```python
from build123d import *

# Parameters (mm, degrees)
SKETCH_1_W                     = 52
SKETCH_1_H                     = 44
EXTRUDE_1_DEPTH                = 7
SKETCH_2_W                     = 40.4
SKETCH_2_H                     = 40.4
CUT_EXTRUDE_1_DEPTH            = 5.5
SKETCH_4_W                     = 7.08
SKETCH_4_H                     = 40.4
EXTRUDE_2_DEPTH                = 1
SKETCH_5_W                     = 5.8
SKETCH_5_H                     = 25.6
CUT_EXTRUDE_2_DEPTH            = 1
SKETCH_7_R                     = 1
CUT_EXTRUDE_3_DEPTH            = 63.531991812
EXTRUDE_3_REACH                = 64.682
SKETCH_13_R                    = 1.75
HOLE_WIZARD_M1_6_1_D           = 1.8
HOLE_WIZARD_M1_6_1_CBORE_D     = 2.6
HOLE_WIZARD_M1_6_1_CBORE_DEPTH = 0.8
CHAMFER_1_SIZE                 = 5.5
CUT_EXTRUDE_4_DEPTH            = 1.6
SKETCH_15_W                    = 10
SKETCH_15_H                    = 12.713519239
CUT_EXTRUDE_5_DEPTH            = 5
CHAMFER_2_SIZE                 = 0.6
FILLET_1_R                     = 1
SKETCH_19_R                    = 0.9
CUT_EXTRUDE_9_DEPTH            = 1.6


with BuildPart() as part:
    # 스케치1 → 보스-돌출1 (new body)
    with BuildSketch(Plane(origin=(0, 7, 0), x_dir=(1, 0, 0), z_dir=(0, 1, 0))):
        with Locations((20, 20)):
            Rectangle(SKETCH_1_W, SKETCH_1_H)
    extrude(amount=-EXTRUDE_1_DEPTH)

    # 스케치2 → 컷-돌출1 (cut)
    with BuildSketch(Plane.XZ):
        with Locations((20, -20)):
            Rectangle(SKETCH_2_W, SKETCH_2_H)
    extrude(amount=-CUT_EXTRUDE_1_DEPTH, mode=Mode.SUBTRACT)

    # 스케치4 → 보스-돌출2 (add)
    # profile 1 of 2: a face of its own
    with BuildSketch(Plane.XZ.offset(-5.5)):
        with Locations((3.34, -20)):
            Rectangle(SKETCH_4_W, SKETCH_4_H)
        with BuildLine():
            Line((4.64, -5), (4.64, -15))
            ThreePointArc((4.64, -15), (3.34, -16.3), (2.04, -15))
            Line((2.04, -15), (2.04, -5))
            ThreePointArc((2.04, -5), (3.34, -3.7), (4.64, -5))
        make_face(mode=Mode.SUBTRACT)
        with BuildLine():
            Line((4.64, -25), (4.64, -35))
            ThreePointArc((4.64, -35), (3.34, -36.3), (2.04, -35))
            Line((2.04, -35), (2.04, -25))
            ThreePointArc((2.04, -25), (3.34, -23.7), (4.64, -25))
        make_face(mode=Mode.SUBTRACT)
    # profile 2 of 2: a face of its own
    with BuildSketch(Plane.XZ.offset(-5.5)):
        with Locations((36.66, -20)):
            Rectangle(SKETCH_4_W, SKETCH_4_H)
        with BuildLine():
            Line((37.96, -5), (37.96, -15))
            ThreePointArc((37.96, -15), (36.66, -16.3), (35.36, -15))
            Line((35.36, -15), (35.36, -5))
            ThreePointArc((35.36, -5), (36.66, -3.7), (37.96, -5))
        make_face(mode=Mode.SUBTRACT)
        with BuildLine():
            Line((35.36, -35), (35.36, -25))
            ThreePointArc((35.36, -25), (36.66, -23.7), (37.96, -25))
            Line((37.96, -25), (37.96, -35))
            ThreePointArc((37.96, -35), (36.66, -36.3), (35.36, -35))
        make_face(mode=Mode.SUBTRACT)
    extrude(amount=EXTRUDE_2_DEPTH)

    # 스케치5 → 컷-돌출2 (cut)
    with BuildSketch(Plane.XZ):
        with Locations((43.1, -20)):
            Rectangle(SKETCH_5_W, SKETCH_5_H)
        with Locations((-3.1, -20)):
            Rectangle(SKETCH_5_W, SKETCH_5_H)
    extrude(amount=-CUT_EXTRUDE_2_DEPTH, mode=Mode.SUBTRACT)

    # 스케치7 → 컷-돌출3 (cut, through all)
    with BuildSketch(Plane.XZ.offset(-5.5)):
        with Locations(Location((28.92, -37.4, 0), (0, 0, 270))):
            Circle(SKETCH_7_R)
        with Locations(Location((11.08, -37.4, 0), (0, 0, 270))):
            Circle(SKETCH_7_R)
    extrude(amount=-CUT_EXTRUDE_3_DEPTH, mode=Mode.SUBTRACT)

    # 스케치13 → 보스-돌출3 (add, up to next)
    with BuildSketch(Plane.XZ, mode=Mode.PRIVATE) as extrude_3_sk1:
        with Locations((7.5, 0)):
            Circle(SKETCH_13_R)
    extrude_3_tool1 = extrude(extrude_3_sk1.sketch, amount=-EXTRUDE_3_REACH, mode=Mode.PRIVATE) - part.part
    # 스케치13 → 보스-돌출3 (add, up to next)
    with BuildSketch(Plane.XZ, mode=Mode.PRIVATE) as extrude_3_sk2:
        with Locations((32.5, 0)):
            Circle(SKETCH_13_R)
    extrude_3_tool2 = extrude(extrude_3_sk2.sketch, amount=-EXTRUDE_3_REACH, mode=Mode.PRIVATE) - part.part
    # 스케치13 → 보스-돌출3 (add, up to next)
    with BuildSketch(Plane.XZ, mode=Mode.PRIVATE) as extrude_3_sk3:
        with Locations((32.5, -40)):
            Circle(SKETCH_13_R)
    extrude_3_tool3 = extrude(extrude_3_sk3.sketch, amount=-EXTRUDE_3_REACH, mode=Mode.PRIVATE) - part.part
    # 스케치13 → 보스-돌출3 (add, up to next)
    with BuildSketch(Plane.XZ, mode=Mode.PRIVATE) as extrude_3_sk4:
        with Locations((7.5, -40)):
            Circle(SKETCH_13_R)
    extrude_3_tool4 = extrude(extrude_3_sk4.sketch, amount=-EXTRUDE_3_REACH, mode=Mode.PRIVATE) - part.part
    add(extrude_3_tool1.solids().sort_by_distance((7.5, 0, 0))[0])
    add(extrude_3_tool2.solids().sort_by_distance((32.5, 0, 0))[0])
    add(extrude_3_tool3.solids().sort_by_distance((32.5, 0, -40))[0])
    add(extrude_3_tool4.solids().sort_by_distance((7.5, 0, -40))[0])

    # M1.6 남비 머리 나사용 카운터보어1 (through all)
    with Locations(Plane(origin=(0, 7, 0), x_dir=(1, 0, 0), z_dir=(0, 1, 0))):
        with Locations((7.5, 0), (32.5, 0), (7.5, 40), (32.5, 40)):
            CounterBoreHole(HOLE_WIZARD_M1_6_1_D / 2, HOLE_WIZARD_M1_6_1_CBORE_D / 2, HOLE_WIZARD_M1_6_1_CBORE_DEPTH)

    # 모따기1
    chamfer_1_edges = [part.edges().sort_by_distance(p)[0] for p in [
        (46, 7, -20),
        (-6, 7, -20),
    ]]
    chamfer(chamfer_1_edges, length=CHAMFER_1_SIZE)

    # 스케치14 → 컷-돌출4 (cut)
    with BuildSketch(Plane.XZ):
        with BuildLine():
            Line((34.238533865, 0.2), (30.761466135, 0.2))
            ThreePointArc((30.761466135, 0.2), (32.5, -1.75), (34.238533865, 0.2))
        make_face()
        with BuildLine():
            Line((9.238533865, 0.2), (5.761466135, 0.2))
            ThreePointArc((5.761466135, 0.2), (7.5, -1.75), (9.238533865, 0.2))
        make_face()
        with BuildLine():
            Line((9.238533865, -40.2), (5.761466135, -40.2))
            ThreePointArc((5.761466135, -40.2), (7.5, -38.25), (9.238533865, -40.2))
        make_face()
        with BuildLine():
            Line((34.238533865, -40.2), (30.761466135, -40.2))
            ThreePointArc((30.761466135, -40.2), (32.5, -38.25), (34.238533865, -40.2))
        make_face()
    extrude(amount=-CUT_EXTRUDE_4_DEPTH, mode=Mode.SUBTRACT)

    # 스케치15 → 컷-돌출5 (cut)
    with BuildSketch(Plane.XZ):
        with Locations((20, -41.191132848)):
            Rectangle(SKETCH_15_W, SKETCH_15_H)
    extrude(amount=-CUT_EXTRUDE_5_DEPTH, mode=Mode.SUBTRACT)

    # 모따기2
    chamfer_2_edges = [part.edges().sort_by_distance(p)[0] for p in [
        (46, 0.75, 2),
        (46, 0.75, -42),
        (-6, 0.75, -42),
        (20, 7, 2),
        (20, 7, -42),
        (-6, 0.75, 2),
    ]]
    chamfer(chamfer_2_edges, length=CHAMFER_2_SIZE)

    # 필렛1
    fillet_1_edges = [part.edges().sort_by_distance(p)[0] for p in [
        (6.88, 5, -1.636490147),
        (9.238533865, 3.55, 0.2),
        (34.238533865, 3.05, 0.2),
        (33.12, 5, -1.636490147),
        (33.12, 5, -38.363509853),
        (30.761466135, 3.55, -40.2),
        (6.88, 5, -38.363509853),
        (5.761466135, 3.05, -40.2),
        (34.238533865, 3.05, -40.2),
        (9.238533865, 3.55, -40.2),
        (30.761466135, 3.55, 0.2),
        (5.761466135, 3.05, 0.2),
        (-0.2, 2.25, -40.2),
        (-0.2, 2.25, 0.2),
        (40.2, 2.25, -40.2),
        (40.2, 2.25, 0.2),
    ]]
    fillet(fillet_1_edges, radius=FILLET_1_R)

    # 스케치19 → 컷-돌출9 (cut)
    with BuildSketch(Plane.XZ):
        with Locations((-0.2, -40.2)):
            Circle(SKETCH_19_R)
        with Locations((-0.2, 0.2)):
            Circle(SKETCH_19_R)
        with Locations((40.2, 0.2)):
            Circle(SKETCH_19_R)
        with Locations((40.2, -40.2)):
            Circle(SKETCH_19_R)
    extrude(amount=-CUT_EXTRUDE_9_DEPTH, mode=Mode.SUBTRACT)


solid = part.part
```
The listing builds one solid part. Answer for the finished solid, in the listing's coordinates (mm). A direction names the side the tool comes from. Round coordinates to 2 decimals unless told otherwise and drop trailing zeros. Write each loop counter-clockwise with the first axis right and the second up, starting at its lowest first coordinate (ties: lowest second). Pieces come first, ordered by that corner, then holes. Notation, with made-up numbers: (-33, 62) -> (14, 62) arc R21 cw to (14, 84) -> close; hole circle Ø2 at (87, -6). An arc over 180 degrees is marked (long way). Answer as a JSON object with one key per item and string values. Group by question number.
Q1. Section A-A (x = 11.08) is taken. Write down the section's boundary in (y, z).
Q2. Each of these flat-tipped pins is pushed along its axis until it touches: pin 1 Ø0.5 at (x, z) = (0, 0.5) entering from -Y; pin 2 Ø1.4 at (x, z) = (19, -40.5) entering from -Y; pin 3 Ø1.1 at (x, z) = (7.5, -40) entering from +Y; pin 4 Ø0.8 at (y, z) = (5, -12) entering from -X. Where does it stop, or does it pass through?
Q3. Section C-C (x = 18.5) is taken. Write down the section's boundary in (y, z), plus the area to 3 significant figures.
Q4. Which of the six approach directions +Z, -Z, +X, -X, +Y, -Y give full straight-line access (tool end or side, diameter ignored) to faces 3 (the face through (25, 2, -41)), 4 (the face through (32.62, 3.06, -40.89)), 5 (the face through (40.857, 0.789, 0.815))?
Q5. Straight lines are drawn through the part: line 1 along Z through (x, y) = (7.5, 4); line 2 along X through (y, z) = (5.95, -37.4); line 3 along Z through (x, y) = (25.5, 1.5). For each, find the intervals that lie inside material, in ascending order.
Q6. Determine the mould class of faces 1 (the face through (20, 0, 1)), 2 (the face through (40.4, 1.6, -40.4)) for opening direction X: pulls with the +X half, pulls with the -X half, needs draft (parallel to the pull), parting line crosses it, or undercut.
Q7. Section D-D (y = 3.5) is taken. Count the separate pieces of the cut face and the enclosed holes in it, plus the area to 3 significant figures.
Q8. Section B-B (z = -20) is taken. Write down the section's boundary in (x, y), plus the area to 3 significant figures.
Check values:
{
 "1": {"outline": "(0, -42) -> (6.4, -42) -> (7, -41.4) -> (7, -38.4) -> (5.5, -38.4) -> (5.5, -40.2) -> (0, -40.2) -> close; (0, 0.2) -> (5.5, 0.2) -> (5.5, -36.4) -> (7, -36.4) -> (7, 1.4) -> (6.4, 2) -> (0, 2) -> close"},
 "2": {"pin 1": "y = 1.6", "pin 2": "y = 5", "pin 3": "through", "pin 4": "x = -2.9"},
 "3": {"outline": "(0, 0.2) -> (5.5, 0.2) -> (5.5, -40.2) -> (5, -40.2) -> (5, -42) -> (6.4, -42) -> (7, -41.4) -> (7, 1.4) -> (6.4, 2) -> (0, 2) -> close", "area": "76.4 mm^2"},
 "4": {"face 3": "-Z, -Y", "face 4": "+Y, -Y", "face 5": "-Y"},
 "5": {"line 1": "-42 to -40.9, -39.1 to -38.25, -1.75 to -0.9, 0.9 to 2", "line 2": "-1.55 to 10.08, 12.08 to 27.92, 29.92 to 41.55", "line 3": "-42 to -40.2, 0.2 to 2"},
 "6": {"face 1": "needs draft", "face 2": "undercut"},
 "7": {"separate pieces": "1", "enclosed holes": "4", "area": "476 mm^2"},
 "8": {"outline": "(-6, 1) -> (-0.2, 1) -> (-0.2, 4.5) -> (6.88, 4.5) -> (6.88, 5.5) -> (33.12, 5.5) -> (33.12, 4.5) -> (40.2, 4.5) -> (40.2, 1) -> (46, 1) -> (46, 1.5) -> (40.5, 7) -> (-0.5, 7) -> (-6, 1.5) -> close", "area": "114 mm^2"}
}
